Read the model definition and answer for the solid it produces. Units are mm, in the model's axes. Round coordinates to 2 decimals unless told otherwise and drop trailing zeros. Order: outer loops, then holes, each group sorted by start corner. A loop starts at its lowest first (then second) coordinate and runs counter-clockwise, first axis right, second up. Notation, with made-up numbers: (-7, 25.25) -> (10, 25.25) arc R21 cw to (10, 63.25) -> close; hole circle Ø1 at (40, 52). An arc over 180 degrees is marked (long way). Use a Markdown table: item, result. Add a question column.
1. Consider L1, parallel to Z at x = -0.5, y = 0; L2, parallel to X at y = 1.5, z = -37; L3, parallel to Z at x = 35.5, y = 0. Determine where each line is inside the solid, lowest interval first. Write a range as [from, to].
2. Section A-A, the plane x = 0 is taken. Give the vertices of the cut face in (y, z).
3. Section D-D, the plane y = 5 is taken. Give the number of separate pieces and of enclosed holes in the cut face, then the cut area to 3 significant figures.
4. Section B-B, the plane z = 0 is taken. Give the vertices of the cut face in (x, y), then the cut area to 3 significant figures.
5. Given pin 1 (1 mm diameter, centred on x = 21.5, y = -3.5, fed in from +Z); pin 2 (6 mm diameter, centred on y = 3.5, z = 25.5, fed in from +X); pin 3 (3 mm diameter, centred on y = -3, z = -12, fed in from -X), each flat-ended and moving along its own axis, determine where each tip first touches the part or whether it passes through.
6. Section C-C, the plane x = -54.5 is taken. Give the vertices of the cut face in (y, z), then the cut area to 3 significant figures.
```python
from build123d import *

# Parameters (mm, degrees)
F0_R     = 72
F0_R_2   = 5
F1_DEPTH = 7.5


with BuildPart() as f1:
    # F0 (on Front) → F1 (new body, symmetric)
    with BuildSketch(Plane.XZ):
        Circle(F0_R)
        with Locations((-38.53732, -38.53732)):
            Circle(F0_R_2, mode=Mode.SUBTRACT)
        with Locations((0, -54.5)):
            Circle(F0_R_2, mode=Mode.SUBTRACT)
        with Locations((38.53732, -38.53732)):
            Circle(F0_R_2, mode=Mode.SUBTRACT)
        with Locations((-54.5, 0)):
            Circle(F0_R_2, mode=Mode.SUBTRACT)
        with Locations((-38.53732, 38.53732)):
            Circle(F0_R_2, mode=Mode.SUBTRACT)
        with Locations((54.5, 0)):
            Circle(F0_R_2, mode=Mode.SUBTRACT)
        with Locations((0, 54.5)):
            Circle(F0_R_2, mode=Mode.SUBTRACT)
        with Locations((38.53732, 38.53732)):
            Circle(F0_R_2, mode=Mode.SUBTRACT)
    extrude(amount=F1_DEPTH, both=True)


solid = f1.part
```
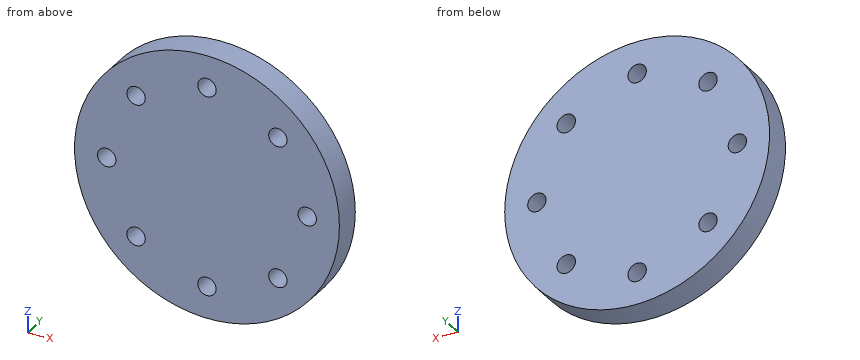
Verdict:
| question | item | result |
|---|---|---|
| 1 | L1 | z = [-72, -59.47], [-49.53, 49.53], [59.47, 72] |
| 1 | L2 | x = [-61.77, -43.3], [-33.78, 33.78], [43.3, 61.77] |
| 1 | L3 | z = [-62.64, -42.51], [-34.57, 34.57], [42.51, 62.64] |
| 2 | outline | (-7.5, -72) -> (7.5, -72) -> (7.5, -59.5) -> (-7.5, -59.5) -> close; (-7.5, -49.5) -> (7.5, -49.5) -> (7.5, 49.5) -> (-7.5, 49.5) -> close; (-7.5, 59.5) -> (7.5, 59.5) -> (7.5, 72) -> (-7.5, 72) -> close |
| 3 | separate pieces | 1 |
| 3 | enclosed holes | 8 |
| 3 | area | 15,700 mm2 |
| 4 | outline | (-72, -7.5) -> (-59.5, -7.5) -> (-59.5, 7.5) -> (-72, 7.5) -> close; (-49.5, -7.5) -> (49.5, -7.5) -> (49.5, 7.5) -> (-49.5, 7.5) -> close; (59.5, -7.5) -> (72, -7.5) -> (72, 7.5) -> (59.5, 7.5) -> close |
| 4 | area | 1,860 mm2 |
| 5 | pin 1 | stops at z = 68.87 |
| 5 | pin 2 | stops at x = 68.39 |
| 5 | pin 3 | stops at x = -71.23 |
| 6 | outline | (-7.5, -47.05) -> (7.5, -47.05) -> (7.5, -5) -> (-7.5, -5) -> close; (-7.5, 5) -> (7.5, 5) -> (7.5, 47.05) -> (-7.5, 47.05) -> close |
| 6 | area | 1,260 mm2 |
